Here's how the part is built. I have some questions about the finished solid (model axes, mm). A direction names the side the tool comes from. Coordinates: 2 decimals unless noted, no trailing zeros. Loops run counter-clockwise (first coordinate to the right, second up) from the corner with the lowest first, then second, coordinate; pieces in that order, holes last. Notation, with made-up numbers: (68.25, -25) -> (117.25, -25) arc R32 cw to (117.25, 9) -> close; hole circle Ø11 at (35, 27). An arc over 180 degrees is marked (long way). Answer as a JSON object with one key per item and string values. Group by question number.
Q1. On a 3-axis mill with a long thin cutter (end or side, diameter ignored), from which of +Z, -Z, +X, -X, +Y, -Y can I reach the whole of each face in a straight line? I mean faces 1 (the flat face through (0.455, -1.933, 0.111)), 2 (the flat face through (-1.933, -0.455, 0.111)), 3 (the cylindrical face through (-1.627, -1.606, 3.87)), 4 (the cylindrical face through (1.606, -1.627, -3.87)). Say none if no direction works.
Q2. I want a section at A-A on z = 5. Write out the boundary of the cut face in (x, y).
Q3. I'm going to push flat-ended pins straight in: pin 1 (0.8 mm diameter, centred on x = -1.5, y = 2, fed in from +Z); pin 2 (0.5 mm diameter, centred on x = -2, y = -1.5, fed in from -Z). Where does each tip first touch, or does it pass through?
Q4. Thinking about a two-plate mould opening in Y: for faces 5 (the flat face through (-1.92, 0.44, 0.11)), 6 (the cylindrical face through (-1.785, -1.807, 0.051)), 7 (the cylindrical face through (-1.606, 1.627, -3.87)), which applies, released by +Y, released by -Y, zero draft, split by the parting line, or undercut?
Q5. I want a section at B-B on x = -0.35. Write out the boundary of the cut face in (y, z), then the cut area to 3 significant figures.
Q6. I need wall thicknesses on line 1 (Y direction, x = -1.6, z = -4.25); line 2 (Y direction, x = 1.65, z = 2); line 3 (X direction, y = 2.05, z = 3). Which ranges of each line are inside material? Lowest first, please.
```python
from build123d import *

# Parameters (mm, degrees)
BOSS_EXTRUDE1_DEPTH = 7.9375
SKETCH2_W           = 0.508
SKETCH2_H           = 0.254
FILLET3_R           = 0.508


with BuildPart() as part:
    # Sketch1 → Boss-Extrude1 (new body, symmetric)
    with BuildSketch(Plane.XY):
        with BuildLine():
            Line((-0.898025612, 2.375952441), (0, 1.477926828))
            Line((0, 1.477926828), (0.898025612, 2.375952441))
            ThreePointArc((0.898025612, 2.375952441), (1.796051224, 1.796051224), (2.375952441, 0.898025612))
            Line((2.375952441, 0.898025612), (1.477926828, 0))
            Line((1.477926828, 0), (2.375952441, -0.898025612))
            ThreePointArc((2.375952441, -0.898025612), (1.796051224, -1.796051224), (0.898025612, -2.375952441))
            Line((0.898025612, -2.375952441), (0, -1.477926828))
            Line((0, -1.477926828), (-0.898025612, -2.375952441))
            ThreePointArc((-0.898025612, -2.375952441), (-1.796051224, -1.796051224), (-2.375952441, -0.898025612))
            Line((-2.375952441, -0.898025612), (-1.477926828, 0))
            Line((-1.477926828, 0), (-2.375952441, 0.898025612))
            ThreePointArc((-2.375952441, 0.898025612), (-1.796051224, 1.796051224), (-0.898025612, 2.375952441))
        make_face()
    extrude(amount=BOSS_EXTRUDE1_DEPTH, both=True)

    # Sketch2 → Cut-Revolve2 (revolve, cut)
    with BuildSketch(Plane(origin=(0, 0, 0), x_dir=(0, 0, -1), z_dir=(1, 0, 0))):
        with Locations((-3.8735, 2.413)):
            Rectangle(SKETCH2_W, SKETCH2_H)
    cut_revolve2 = revolve(axis=Axis((0, 0, 0), (0, 0, 1)), mode=Mode.SUBTRACT)

    # Mirror1: Cut-Revolve2 across plane
    add(cut_revolve2.mirror(Plane.XY), mode=Mode.SUBTRACT)

    # Fillet3
    fillet3_edges = [part.edges().sort_by_distance(p)[0] for p in [
        (1.796051224, 1.796051224, -7.9375),
        (1.796051224, -1.796051224, -7.9375),
        (-1.796051224, -1.796051224, -7.9375),
        (-1.796051224, 1.796051224, -7.9375),
        (-1.796051224, -1.796051224, 7.9375),
        (1.796051224, -1.796051224, 7.9375),
        (1.796051224, 1.796051224, 7.9375),
        (-1.796051224, 1.796051224, 7.9375),
    ]]
    fillet(fillet3_edges, radius=FILLET3_R)


solid = part.part
```
Result set:
{
 "1": {"face 1": "+Z, -Z, -Y", "face 2": "+Z, -Z, -X", "face 3": "-X, -Y", "face 4": "+X, -Y"},
 "2": {"outline": "(-2.38, -0.9) arc R2.54 ccw to (-0.9, -2.38) -> (0, -1.48) -> (0.9, -2.38) arc R2.54 ccw to (2.38, -0.9) -> (1.48, 0) -> (2.38, 0.9) arc R2.54 ccw to (0.9, 2.38) -> (0, 1.48) -> (-0.9, 2.38) arc R2.54 ccw to (-2.38, 0.9) -> (-1.48, 0) -> close"},
 "3": {"pin 1": "stops at z = 7.93", "pin 2": "stops at z = -7.89"},
 "4": {"face 5": "undercut", "face 6": "released by -Y", "face 7": "released by +Y"},
 "5": {"outline": "(-1.83, -7.94) -> (1.83, -7.94) -> (1.83, 7.94) -> (-1.83, 7.94) -> close", "area": "58.0 mm²"},
 "6": {"line 1": "y = -1.97 to -0.12, 0.12 to 1.97", "line 2": "y = -1.93 to -0.17, 0.17 to 1.93", "line 3": "x = -1.5 to -0.57, 0.57 to 1.5"}
}
